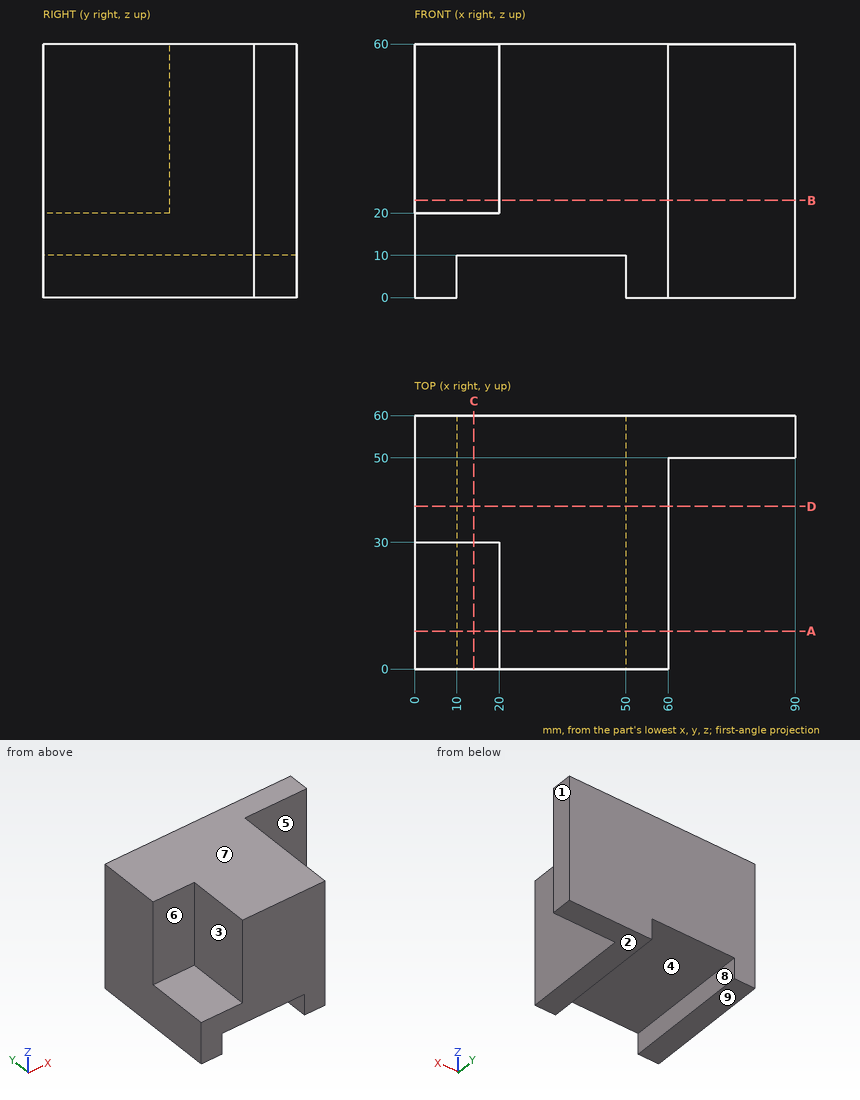
Geometry: see drawing. Coordinates: mm, zero at the bounding-box minimum. A direction names the side the tool comes from. Coordinates: 2 decimals unless noted, no trailing zeros. Loops run counter-clockwise (first coordinate to the right, second up) from the corner with the lowest first, then second, coordinate; pieces in that order, holes last.
(1) Pull-direction query (X, two-part tool) for the marked faces 1, 2, 3 and 4; classes: released by +X, released by -X, zero draft, split by the parting line, or undercut.
(2) Section D-D on y = 38.5. Return the cut outline in (x, z), then the cut area to 3 significant figures.
(3) First-contact query: pin 1 Ø2 at (x, z) = (20.5, 42.5) entering from -Y; pin 2 Ø24 at (x, z) = (74, 39) entering from -Y; pin 3 Ø3 at (x, y) = (13.5, 17) entering from +Z; pin 4 Ø10 at (x, z) = (9.5, 42) entering from -Y. Flat tips, straight axial feed; report the tip coordinate or a pass-through.
(4) Section C-C on x = 14. Return the cut outline in (y, z), then the cut area to 3 significant figures.
(5) Section A-A on y = 9. Return the cut outline in (x, z).
(6) Set-up query: the marked faces 5, 6, 7, 8 and 9. Return all of +Z, -Z, +X, -X, +Y, -Y with unobstructed straight access to the full face (end or side cutting, diameter ignored); none if empty.
(7) Material intervals for probe 1 along Z at (x, y) = (45, 9.5); probe 2 along X at (y, z) = (9, 30); probe 3 along X at (y, z) = (27, 5), sorted ascending.
(8) Section B-B on z = 23. Return the cut outline in (x, y), then the cut area to 3 significant figures.
Data:
1. face 1: released by +X
1. face 2: zero draft
1. face 3: released by -X
1. face 4: undercut
2. outline: (0, 0) - (10, 0) - (10, 10) - (50, 10) - (50, 0) - (60, 0) - (60, 60) - (0, 60) - close
2. area: 3,200 mm2
3. pin 1: stops at y = 0
3. pin 2: stops at y = 50
3. pin 3: stops at z = 20
3. pin 4: stops at y = 30
4. outline: (0, 10) - (60, 10) - (60, 60) - (30, 60) - (30, 20) - (0, 20) - close
4. area: 1,800 mm2
5. outline: (0, 0) - (10, 0) - (10, 10) - (50, 10) - (50, 0) - (60, 0) - (60, 60) - (20, 60) - (20, 20) - (0, 20) - close
6. face 5: +Z, -Z, +X, -Y
6. face 6: +Z, -X, -Y
6. face 7: +Z, +X, -X, +Y, -Y
6. face 8: -Z, +Y, -Y
6. face 9: -Z, +X, -X, +Y, -Y
7. probe 1: z = 10 to 60
7. probe 2: x = 20 to 60
7. probe 3: x = 0 to 10, 50 to 60
8. outline: (0, 30) - (20, 30) - (20, 0) - (60, 0) - (60, 50) - (90, 50) - (90, 60) - (0, 60) - close
8. area: 3,300 mm2
